Build history of the part. All positions in model axes, mm. A direction names the side the tool comes from. Give positions to 0.01 mm unless a question says otherwise; leave off trailing zeros. Order: outer loops, then holes, each group sorted by start corner. A loop starts at its lowest first (then second) coordinate and runs counter-clockwise, first axis right, second up. Notation, with made-up numbers: (88.5, -13.75) - (139.5, -13.75) arc R20 ccw to (139.5, -4.75) - close; hole circle Ø3 at (89, 74.25). An arc over 180 degrees is marked (long way). Write each question's results on one line, items separated by ' | '. Start each with the question number.
from build123d import *

# Parameters (mm, degrees)
SKETCH_1_R          = 12.5
EXTRUDE_1_DEPTH     = 17
SKETCH_2_R          = 16
EXTRUDE_2_DEPTH     = 51
SKETCH_3_R          = 2
EXTRUDE_3_DEPTH     = 8.8
SKETCH_7_R          = 20.782497367
SKETCH_7_R_2        = 13.5
CUT_EXTRUDE_8_DEPTH = 4


with BuildPart() as part:
    # Эскиз1 → Вытянуть1 (new body)
    with BuildSketch(Plane.XY):
        Circle(SKETCH_1_R)
    extrude(amount=EXTRUDE_1_DEPTH)

    # Эскиз2 → Вытянуть2 (add)
    with BuildSketch(Plane.XY.offset(17)):
        Circle(SKETCH_2_R)
    extrude(amount=EXTRUDE_2_DEPTH)

    # Эскиз3 → Вытянуть3 (add)
    with BuildSketch(Plane.XY.offset(68)):
        Circle(SKETCH_3_R)
    extrude(amount=EXTRUDE_3_DEPTH)

    # Эскиз7 → Вытянуть8 (cut)
    with BuildSketch(Plane.XY.offset(38)):
        Circle(SKETCH_7_R)
        Circle(SKETCH_7_R_2, mode=Mode.SUBTRACT)
    extrude(amount=CUT_EXTRUDE_8_DEPTH, mode=Mode.SUBTRACT)


solid = part.part
Item 1: Cut at C-C, the plane z = 48. List the corners of the cut face in (x, y).
Item 2: Probe line 1 along Z through (x, y) = (-1, 14.5); line 2 along Z through (x, y) = (6.5, -6.5); line 3 along Z through (x, y) = (-8, -10). List the from-to ranges inside material, lowest first. Write a range as from..to.
Item 3: Which spindle directions (+Z, -Z, +X, -X, +Y, -Y) get a long thin tool onto all of the face, cutting with end or side? Do faces 1 (the cylindrical face through (0, -2, 72)), 2 (the flat face through (-7, -12, 42)), 3 (the cylindrical face through (-3.47, -15.62, 27.35)), 4 (the flat face through (0, 0, 0)), 5 (the cylindrical face through (11.923, 3.755, 8.381)). Say none if no direction does.
Item 4: Two-plate mould, pull along Z, no slides. Class faces 6 (the flat face through (-10, -8, 17)), 7 (the flat face through (0, 0, 76.8)), 8 (the flat face through (-7, -12, 38)), 9 (the cylindrical face through (-2.93, -13.18, 39.97)): +Z half, -Z half, draft (parallel to the pull), parting line (faces both ways), or undercut.
Item 5: Cut at A-A, the plane x = 0. List the corners of the cut face in (y, z).
Item 6: Flat gauge pins, fed straight in: pin 1 Ø1.5 at (x, y) = (-9, -12) entering from -Z; pin 2 Ø5 at (x, y) = (-12, -4.5) entering from +Z; pin 3 Ø2 at (x, z) = (-12, 33) entering from -Y. Where does each tip first touch, or does it go through?
Item 7: Cut at D-D, the plane x = -7.5. List the corners of the cut face in (y, z).
Values found:
1) outline: circle Ø32 at (0, 0)
2) line 1: z = 17..38, 42..68 | line 2: z = 0..68 | line 3: z = 17..68
3) face 1: +Z | face 2: none | face 3: +Z, -Z | face 4: -Z, +X, -X, +Y, -Y | face 5: -Z
4) face 6: -Z half | face 7: +Z half | face 8: undercut | face 9: undercut
5) outline: (-16, 17) - (-12.5, 17) - (-12.5, 0) - (12.5, 0) - (12.5, 17) - (16, 17) - (16, 38) - (13.5, 38) - (13.5, 42) - (16, 42) - (16, 68) - (2, 68) - (2, 76.8) - (-2, 76.8) - (-2, 68) - (-16, 68) - (-16, 42) - (-13.5, 42) - (-13.5, 38) - (-16, 38) - close
6) pin 1: stops at z = 17 | pin 2: stops at z = 68 | pin 3: stops at y = -11.62
7) outline: (-14.13, 17) - (-10, 17) - (-10, 0) - (10, 0) - (10, 17) - (14.13, 17) - (14.13, 38) - (11.22, 38) - (11.22, 42) - (14.13, 42) - (14.13, 68) - (-14.13, 68) - (-14.13, 42) - (-11.22, 42) - (-11.22, 38) - (-14.13, 38) - close
